```python
from build123d import *

# Parameters (mm, degrees)
BOSS_EXTRUDE1_DEPTH = 4
SKETCH1_3_R         = 1.5
SKETCH1_3_R_2       = 2
BOSS_EXTRUDE2_DEPTH = 9
FILLET1_R           = 0.5


with BuildPart() as part:
    # Sketch1 → Boss-Extrude1 (new body)
    with BuildSketch(Plane.XY):
        with BuildLine():
            Line((0, 0), (0, -4))
            Line((0, -4), (37.08, -4))
            Line((37.08, -4), (37.08, 0))
            ThreePointArc((37.08, 0), (18.54, 2.327664136), (0, 0))
        make_face()
    extrude(amount=BOSS_EXTRUDE1_DEPTH)

    # Sketch1<3> → Boss-Extrude2 (add)
    with BuildSketch(Plane.XY):
        with Locations((1.5, -2)):
            Circle(SKETCH1_3_R)
        with Locations((35.08, -2)):
            Circle(SKETCH1_3_R_2)
    extrude(amount=-BOSS_EXTRUDE2_DEPTH)

    # Fillet1
    fillet1_edges = [part.edges().sort_by_distance(p)[0] for p in [
        (37.08, 0, 2),
        (37.08, -4, 2),
        (0, -4, 2),
        (0, 0, 2),
    ]]
    fillet(fillet1_edges, radius=FILLET1_R)


solid = part.part
```
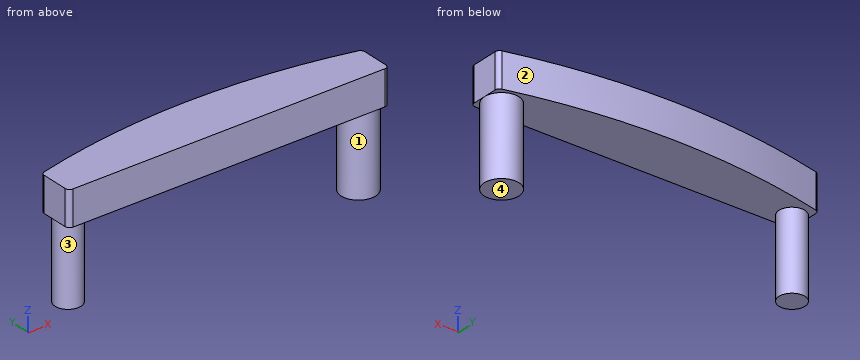
Work out the finished part from the listing and answer in its coordinate system (mm). Face numbers are marked on the shaded views. Coordinates: 2 decimals unless noted, no trailing zeros. Loops run counter-clockwise (first coordinate to the right, second up) from the corner with the lowest first, then second, coordinate; pieces in that order, holes last. Notation, with made-up numbers: (25.25, 47) - (63.25, 47) arc R23 ccw to (63.25, 55) - close; hole circle Ø6 at (26, -37). An arc over 180 degrees is marked (long way). Use a Markdown table: item, result.
Item 1: Find section D-D, the plane y = -1. Determine the outline of the cut face in (x, z), and give its area (3 significant figures).
Evaluation:
| item | result |
|---|---|
| outline | (0, 0) - (0.38, 0) - (0.38, -9) - (2.62, -9) - (2.62, 0) - (33.35, 0) - (33.35, -9) - (36.81, -9) - (36.81, 0) - (37.08, 0) - (37.08, 4) - (0, 4) - close |
| area | 200 mm2 |
Item 2: The mould has two halves that part along X. Classify the marked faces 1, 2, 3 and 4: +X half, -X half, draft (parallel to the pull), parting line (faces both ways), or undercut.
Evaluation:
| item | result |
|---|---|
| face 1 | undercut |
| face 2 | parting line |
| face 3 | undercut |
| face 4 | draft |
Item 3: Find section C-C, the plane y = -2.5. Determine the outline of the cut face in (x, z).
Evaluation:
| item | result |
|---|---|
| outline | (0, 0) - (0.09, 0) - (0.09, -9) - (2.91, -9) - (2.91, 0) - (33.14, 0) - (33.14, -9) - (37.02, -9) - (37.02, 0) - (37.08, 0) - (37.08, 4) - (0, 4) - close |
Item 4: Consider probe 1 along X at (y, z) = (-2, -6.25); probe 2 along Z at (x, y) = (10.5, -2); probe 3 along X at (y, z) = (-1.5, -5.5). Determine where each line is inside the solid, lowest interval first. Write a range as from..to.
Evaluation:
| item | result |
|---|---|
| probe 1 | x = 0..3, 33.08..37.08 |
| probe 2 | z = 0..4 |
| probe 3 | x = 0.09..2.91, 33.14..37.02 |
Item 5: Find section A-A, the plane z = 0.75. Determine the outline of the cut face in (x, y).
Evaluation:
| item | result |
|---|---|
| outline | (0, -3.5) arc R0.5 ccw to (0.5, -4) - (36.58, -4) arc R0.5 ccw to (37.08, -3.5) - (37.08, -0.39) arc R0.5 ccw to (36.7, 0.1) arc R75 ccw to (0.38, 0.1) arc R0.5 ccw to (0, -0.39) - close |
Item 6: Find section B-B, the plane x = 1.5. Determine the outline of the cut face in (y, z), and give its area (3 significant figures).
Evaluation:
| item | result |
|---|---|
| outline | (-4, 0) - (-3.5, 0) - (-3.5, -9) - (-0.5, -9) - (-0.5, 0) - (0.37, 0) - (0.37, 4) - (-4, 4) - close |
| area | 44.5 mm2 |
